Read the model definition and answer for the solid it produces. Units are mm, in the model's axes. A direction names the side the tool comes from. Give positions to 0.01 mm unless a question says otherwise; leave off trailing zeros. Order: outer loops, then holes, each group sorted by start corner. A loop starts at its lowest first (then second) coordinate and runs counter-clockwise, first axis right, second up.
```python
from build123d import *

# Parameters (mm, degrees)
SKETCH1_R               = 14.5
BOSS_EXTRUDE1_DEPTH     = 12.5
CUT_EXTRUDE1_START      = -10
SKETCH2_R               = 14.5
SKETCH2_R_2             = 12
CUT_EXTRUDE1_DEPTH      = 10
SKETCH4_R               = 11
CUT_EXTRUDE2_DEPTH      = 25.015619917
CUT_EXTRUDE3_DEPTH      = 25.015619917
CUT_EXTRUDE3_DEPTH_BACK = 25.015619917


with BuildPart() as part:
    # Sketch1 → Boss-Extrude1 (new body)
    with BuildSketch(Plane(origin=(0, 0, 0), x_dir=(1, 0, 0), z_dir=(0, 1, 0))):
        with Locations(Location((0, 0, 0), (0, 0, 270))):
            Circle(SKETCH1_R)
    extrude(amount=BOSS_EXTRUDE1_DEPTH)

    # Sketch2 → Cut-Extrude1 (cut)
    with BuildSketch(Plane(origin=(0, 12.5, 0), x_dir=(1, 0, 0), z_dir=(0, 1, 0)).offset(CUT_EXTRUDE1_START)):
        with Locations(Location((0, 0, 0), (0, 0, 270))):
            Circle(SKETCH2_R)
        with Locations(Location((0, 0, 0), (0, 0, 270))):
            Circle(SKETCH2_R_2, mode=Mode.SUBTRACT)
    extrude(amount=CUT_EXTRUDE1_DEPTH, mode=Mode.SUBTRACT)

    # Sketch4 → Cut-Extrude2 (cut, through all)
    with BuildSketch(Plane(origin=(0, 12.5, 0), x_dir=(1, 0, 0), z_dir=(0, 1, 0))):
        with Locations(Location((0, 0, 0), (0, 0, 270))):
            Circle(SKETCH4_R)
    extrude(amount=-CUT_EXTRUDE2_DEPTH, mode=Mode.SUBTRACT)

    # Sketch5 → Cut-Extrude3 (cut, two sides: drawn at the far end of the back side and taken through both)
    with BuildSketch(Plane.XY.offset(-CUT_EXTRUDE3_DEPTH_BACK)):
        Polygon((-12, 12.5), (12, 12.5), (12, 7.5), align=None)
    extrude(amount=CUT_EXTRUDE3_DEPTH + CUT_EXTRUDE3_DEPTH_BACK, mode=Mode.SUBTRACT)


solid = part.part
```
1) For a pull along Z with two mould halves and no side action, classify faces 3 (the face through (-10.74, 4.87, -2.38)), 4 (the face through (-5.554, 1.232, 13.394)), 5 (the face through (-3.5, 10.73, 10.61)) as released by +Z, released by -Z, zero draft, split by the parting line, or undercut.
Final values:
face 3: undercut
face 4: split by the parting line
face 5: zero draft
2) The part is cut by section C-C on y = 5. Determine the outline of the cut face in (x, z).
Final values:
outline: circle Ø24 at (0, 0); hole circle Ø22 at (0, 0)
3) Given pin 1 (1 mm diameter, centred on x = -4, y = 6.5, fed in from +Z); pin 2 (1.5 mm diameter, centred on y = 7.5, z = -5.5, fed in from -X); pin 3 (8.5 mm diameter, centred on x = -5, z = -6.5, fed in from +Y), each flat-ended and moving along its own axis, determine where each tip first touches the part or whether it passes through.
Final values:
pin 1: stops at z = 11.48
pin 2: stops at x = -11.02
pin 3: stops at y = 11.93
4) The part is cut by section D-D on x = 11.5. Determine the outline of the cut face in (y, z).
Final values:
outline: (0, -8.83) - (2.5, -8.83) - (2.5, -3.43) - (7.6, -3.43) - (7.6, 3.43) - (2.5, 3.43) - (2.5, 8.83) - (0, 8.83) - close
5) Consider L1, parallel to Z at x = 0, y = 8; L2, parallel to X at y = 6.75, z = 8.25. Determine where each line is inside the solid, lowest interval first.
Final values:
L1: z = -12 to -11, 11 to 12
L2: x = -8.71 to -7.28, 7.28 to 8.71
6) A tool of negligible diameter and unlimited length cuts with its end or side. For faces 1 (the face through (11, 0, -2)), 2 (the face through (12, 2.5, 2)), from which of +Z, -Z, +X, -X, +Y, -Y can it reach the whole face along a straight path? Write none if from no direction.
Final values:
face 1: +Z, -Z, +X, -X, -Y
face 2: +Y
7) The part is cut by section A-A on x = 0. Determine the outline of the cut face in (y, z), and give its area (3 significant figures).
Final values:
outline: (0, -14.5) - (2.5, -14.5) - (2.5, -12) - (10, -12) - (10, -11) - (0, -11) - close; (0, 11) - (10, 11) - (10, 12) - (2.5, 12) - (2.5, 14.5) - (0, 14.5) - close
area: 32.5 mm2
8) The part is cut by section B-B on z = 10.5. Determine the outline of the cut face in (x, y).
Final values:
outline: (-10, 0) - (-3.28, 0) - (-3.28, 10.68) - (-5.81, 11.21) - (-5.81, 2.5) - (-10, 2.5) - close; (3.28, 0) - (10, 0) - (10, 2.5) - (5.81, 2.5) - (5.81, 8.79) - (3.28, 9.32) - close
